Input: part model. Units: mm. Frame: model coordinates. Face numbers are marked on the shaded views. Coordinates: 2 decimals unless noted, no trailing zeros. Write each loop counter-clockwise with the first axis right and the second up, starting at its lowest first coordinate (ties: lowest second). Pieces come first, ordered by that corner, then holes. Notation, with made-up numbers: (-30.75, 47) - (-20.75, 47) arc R14 cw to (-20.75, 74) - close; hole circle Ø1 at (48, -14.75). An arc over 180 degrees is marked (long way). Put each result on its own line as item: value. Start each with the question number.
1. Line query: line 1 (Z direction, x = 8.5, y = 4.15); line 2 (X direction, y = 4.1, z = -1); line 3 (Z direction, x = 9.5, y = 4.2). Output: solid intervals per line, ascending.
2. Cut plane A-A, the plane z = 0. Return loops of the section in (x, y), and give its area (3 significant figures).
3. Pull-direction query (Y, two-part tool) for the marked faces 1 and 2; classes: released by +Y, released by -Y, zero draft, split by the parting line, or undercut.
4. Cut plane B-B, the plane y = 4.1. Count the separate pieces of the cut face and the enclosed holes in it, and give its area (3 significant figures).
Autodesk Inventor part; units mm, degrees
ref_plane "YZ Plane" through (0, 0, 0) normal (1, 0, 0) x (0, 1, 0)
ref_plane "XZ Plane" through (0, 0, 0) normal (0, 1, 0) x (-1, 0, 0)
ref_plane "XY Plane" through (0, 0, 0) normal (0, 0, 1) x (1, 0, 0)
sketch "Boceto1" plane through (0, 0, 0) normal (0, 0, 1) x (1, 0, 0)
  line L0 (2.7328, 4.3298) -> (8.5721, 4.3298)
  line L1 (3.0328, 4.0298) -> (8.5721, 4.0298)
  line L2 (8.5721, 4.3298) -> (8.5721, 4.0298)
  line L3 (2.7328, 4.3298) -> (3.0328, 4.0298)
  point P0 (0, 0)
revolve "Revolución1" add sketch "Boceto1" angle 360 about axis through (8.5721, 4.3298, 0) along (0, -1, 0)
sketch "Boceto3" plane through (8.5721, 4.0298, 0) normal (0, -1, 0) x (1, 0, 0)
  circle A0 centre (0, 0) radius 5.5393
  circle A1 centre (0, 0) radius 5.8393
  circle A2 centre (0, 4.7895) radius 0.675
  circle A3 centre (0, -4.7895) radius 0.675
  point P0 (-8.5721, 0)
  point P1 (0, -4.7895)
  dimension "d5" = 1.35
  dimension "d6" = 1.35
extrude "Extrusión2" cut sketch "Boceto3" against normal blind 0.17 contours A2 | A3
sketch "Boceto4" plane through (8.5721, 4.0298, 0) normal (0, -1, 0) x (1, 0, 0)
  circle A0 centre (0, 0) radius 5.5393
  circle A1 centre (0, 0) radius 1.55
  point P0 (-8.5721, 0)
  dimension "d9" = 3.1
extrude "Extrusión3" cut sketch "Boceto4" against normal blind 10 contours A1
properties part number "cuello"
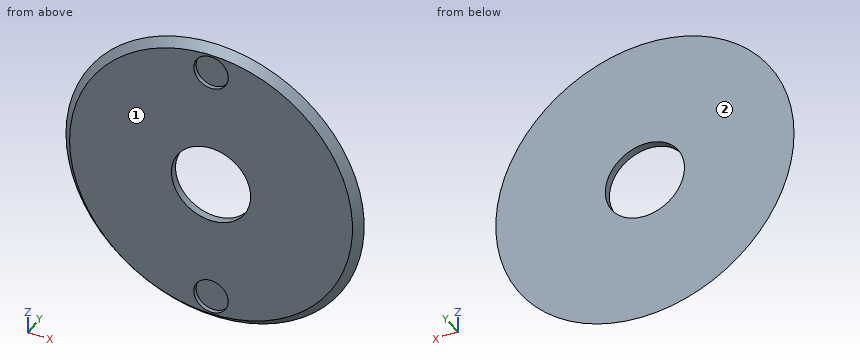
Report:
1. line 1: z = -5.66 to -5.46, -4.12 to -1.55, 1.55 to 4.12, 5.46 to 5.66
1. line 2: x = 3.05 to 7.39, 9.76 to 14.09
1. line 3: z = -5.63 to -1.24, 1.24 to 5.63
2. outline: (2.73, 4.33) - (3.03, 4.03) - (7.02, 4.03) - (7.02, 4.33) - close; (10.12, 4.03) - (14.11, 4.03) - (14.41, 4.33) - (10.12, 4.33) - close
2. area: 2.48 mm^2
3. face 1: released by -Y
3. face 2: released by +Y
4. separate pieces: 1
4. enclosed holes: 3
4. area: 88.4 mm^2
